Part model, mm, in its own coordinate system. Give positions to 0.01 mm unless a question says otherwise; leave off trailing zeros. Order: outer loops, then holes, each group sorted by start corner. A loop starts at its lowest first (then second) coordinate and runs counter-clockwise, first axis right, second up.
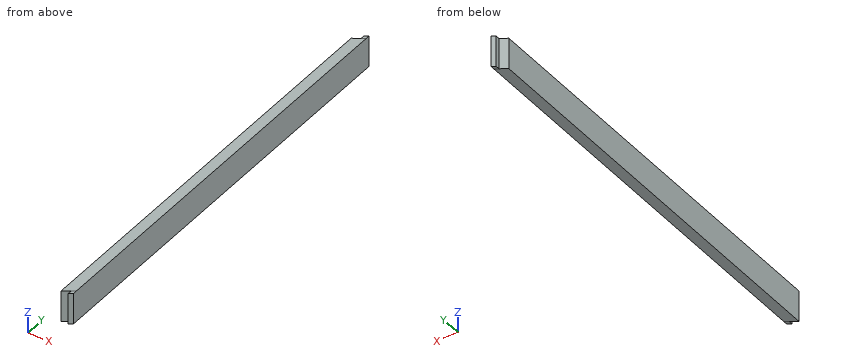
from build123d import *

# Parameters (mm, degrees)
F1_DEPTH = 1056
F3_DEPTH = 10
F5_DEPTH = 10


with BuildPart() as f1:
    # F0 (on Front) → F1 (new body)
    with BuildSketch(Plane.XZ):
        Polygon((0, 79), (0, 0), (38, 15.740115), (38, 94.740115), align=None)
    extrude(amount=-F1_DEPTH)

    # F2 (on face) → F3 (join)
    with BuildSketch(Plane.XZ):
        Polygon((38, 94.740115), (25, 89.355339), (25, 10.355339), (38, 15.740115), align=None)
    extrude(amount=F3_DEPTH)

    # F4 (on face) → F5 (join)
    with BuildSketch(Plane(origin=(0, 1056, 0), x_dir=(-1, 0, 0), z_dir=(0, 1, 0))):
        Polygon((-38, 94.740115), (-38, 15.740115), (-25, 10.355339), (-25, 89.355339), align=None)
    extrude(amount=F5_DEPTH)


solid = f1.part
Item 1: Drop flat-ended pins along their axis: P1, Ø1.5, axis at x = 34, y = 295, coming from the -Z side; P2, Ø5, axis at x = 6, y = 410.5, coming from the -Z side; P3, Ø3, axis at y = 1060.5, z = 48, coming from the -X side. Give the stop position or say it passes through.
Item 2: Drill centre lines: probe 1 along Y at (x, z) = (9, 31.5); probe 2 along Z at (x, y) = (36, 463.5); probe 3 along Z at (x, y) = (18.5, 36.5). Where is each one in solid material? Low to high.
Item 3: Band-saw the part on B-B on x = 31. List the corners of the cut face in (y, z), plus the area to 3 significant figures.
Item 4: Band-saw the part on A-A on y = 286. List the corners of the cut face in (x, z).
Working result:
1. P1: stops at z = 13.77
1. P2: stops at z = 1.45
1. P3: stops at x = 25
2. probe 1: y = 0 to 1056
2. probe 2: z = 14.91 to 93.91
2. probe 3: z = 7.66 to 86.66
3. outline: (-10, 12.84) - (1066, 12.84) - (1066, 91.84) - (-10, 91.84) - close
3. area: 85,000 mm2
4. outline: (0, 0) - (38, 15.74) - (38, 94.74) - (0, 79) - close
